```python
from build123d import *

# Parameters (mm, degrees)
BOX002_W          = 2
BOX002_H          = 4.5
BOX002_DEPTH      = 15.8
CYLINDER001_R     = 6.4
CYLINDER001_DEPTH = 24
CYLINDER_R        = 7.9
CYLINDER_DEPTH    = 24


with BuildPart() as schlitz:
    # Box002 → Box002 (new body)
    with BuildSketch(Plane(origin=(-1, 5.4, 16), x_dir=(1, 0, 0), z_dir=(0, 0, 1))):
        with Locations((1, 2.25)):
            Rectangle(BOX002_W, BOX002_H)
    extrude(amount=BOX002_DEPTH)


with BuildPart() as kegel001:
    # Cone001 → Cone001 (revolve)
    with BuildSketch(Plane(origin=(0, 0, 24), x_dir=(1, 0, 0), z_dir=(0, -1, 0))):
        Polygon((0, 0), (6.4, 0), (2.5, 16.2), (0, 16.2), align=None)
    revolve(axis=Axis((0, 0, 24), (0, 0, 1)))


with BuildPart() as cut001:
    # Cone → Cone (revolve)
    with BuildSketch(Plane(origin=(0, 0, 24), x_dir=(1, 0, 0), z_dir=(0, -1, 0))):
        Polygon((0, 0), (7.9, 0), (4, 16.2), (0, 16.2), align=None)
    revolve(axis=Axis((0, 0, 24), (0, 0, 1)))

    # Cut001: cut Kegel001
    add(kegel001.part, mode=Mode.SUBTRACT)


with BuildPart() as loch_vorne:
    # Cylinder001 → Cylinder001 (new body)
    with BuildSketch(Plane.XY):
        Circle(CYLINDER001_R)
    extrude(amount=CYLINDER001_DEPTH)


with BuildPart() as obj1:
    # Cylinder → Cylinder (new body)
    with BuildSketch(Plane.XY):
        Circle(CYLINDER_R)
    extrude(amount=CYLINDER_DEPTH)

    # Cut: cut Loch_vorne
    add(loch_vorne.part, mode=Mode.SUBTRACT)

    # Fusion001: union Cut001
    add(cut001.part)

    # Cut002: cut Schlitz
    add(schlitz.part, mode=Mode.SUBTRACT)


solid = obj1.part
```
Build history of the part. All positions in model axes, mm. A direction names the side the tool comes from. Coordinates: 2 decimals unless noted, no trailing zeros. Write each loop counter-clockwise with the first axis right and the second up, starting at its lowest first coordinate (ties: lowest second). Pieces come first, ordered by that corner, then holes.
1. Band-saw the part on B-B, the plane x = 0. Give the cut face in (y, z), and give its area (3 significant figures).
Answer block:
outline: (-7.9, 0) - (-6.4, 0) - (-6.4, 24) - (-2.5, 40.2) - (-4, 40.2) - (-7.9, 24) - close; (2.5, 40.2) - (5.4, 28.15) - (5.4, 31.8) - (6.02, 31.8) - (4, 40.2) - close; (6.4, 0) - (7.9, 0) - (7.9, 16) - (6.4, 16) - close
area: 98.5 mm2
2. Pull direction X, two halves, no side cores. Call faces 1 (the flat face through (-1, 7, 24)), 2 (the flat face through (2, 2, 40.2)), 3 (the flat face through (1, 7, 24)), 4 (the cylindrical face through (-6.269, -4.807, 11.832)): released by +X, released by -X, zero draft, split by the parting line, or undercut.
Answer block:
face 1: undercut
face 2: zero draft
face 3: undercut
face 4: split by the parting line
3. Band-saw the part on C-C, the plane z = 8. Give the cut face in (x, y).
Answer block:
outline: circle Ø15.8 at (0, 0); hole circle Ø12.8 at (0, 0)
4. Drill centre lines: probe 1 along X at (y, z) = (0, 18.75); probe 2 along X at (y, z) = (-4, 10). Where is each one in solid material? Low to high.
Answer block:
probe 1: x = -7.9 to -6.4, 6.4 to 7.9
probe 2: x = -6.81 to -5, 5 to 6.81
5. Band-saw the part on D-D, the plane z = 37. Give the cut face in (x, y), and give its area (3 significant figures).
Answer block:
outline: circle Ø9.54 at (0, 0); hole circle Ø6.54 at (0, 0)
area: 37.9 mm2
6. Band-saw the part on A-A, the plane y = 0. Give the cut face in (x, z).
Answer block:
outline: (-7.9, 0) - (-6.4, 0) - (-6.4, 24) - (-2.5, 40.2) - (-4, 40.2) - (-7.9, 24) - close; (2.5, 40.2) - (6.4, 24) - (6.4, 0) - (7.9, 0) - (7.9, 24) - (4, 40.2) - close
7. Drop flat-ended pins along their axis: pin 1 (3 mm diameter, centred on x = -1, y = 2, fed in from +Z); pin 2 (1.5 mm diameter, centred on x = -3, z = 28.5, fed in from +Y); pin 3 (1 mm diameter, centred on y = 1, z = 27.5, fed in from +X); pin 4 (8 mm diameter, centred on x = 0, z = 32, fed in from -Y). Give the stop position or say it passes through.
Answer block:
pin 1: stops at z = 40.2
pin 2: stops at y = 6.5
pin 3: stops at x = 7.12
pin 4: stops at y = -6.94
8. 3-axis set-ups, long thin cutter, end or side, ignore diameter. For faces 5 (the cylindrical face through (-1.387, -6.248, 11.832)), 6 (the conical face through (-1.19, -5.36, 34.01)), 7 (the flat face through (3, -6, 0)), 8 (the flat face through (0, 7, 16)), 9 (the flat face through (0, 5.4, 30)): which of +Z, -Z, +X, -X, +Y, -Y reach the whole face in a straight line?
Answer block:
face 5: -Z
face 6: +Z
face 7: -Z, +X, -X, +Y, -Y
face 8: +Z, +Y
face 9: -Z, +Y
